The listing builds one solid part. Answer for the finished solid, in the listing's coordinates (mm). A direction names the side the tool comes from. Round coordinates to 2 decimals unless told otherwise and drop trailing zeros. Loops run counter-clockwise (first coordinate to the right, second up) from the corner with the lowest first, then second, coordinate; pieces in that order, holes last. Notation, with made-up numbers: (51, 61) -> (55, 61) arc R26 ccw to (55, 93) -> close; hole circle Ø6 at (12.25, 14.25). An arc over 180 degrees is marked (long way). Use a Markdown table: item, result. Add a question column.
Q1. Consider line 1 (Y direction, x = 0.1, z = -63.5); line 2 (Y direction, x = 1.25, z = -109); line 3 (Z direction, x = 1.85, y = -17.5). Determine where each line is inside the solid, lowest interval first.
Q2. Section B-B on y = -16.5 is taken. Give the vertices of the cut face in (x, z).
Q3. Section A-A on z = -14 is taken. Give the vertices of the cut face in (x, y), then the cut area to 3 significant figures.
Q4. For a pull along Y with two mould halves and no side action, classify faces 1 (the flat face through (1, 0, -65)), 2 (the flat face through (1.48, -44.61, -46.78)), 3 (the cylindrical face through (1.521, -11.014, -69.722)) as released by +Y, released by -Y, zero draft, split by the parting line, or undercut.
Q5. Which of the six approach directions +Z, -Z, +X, -X, +Y, -Y give full straight-line access (tool end or side, diameter ignored) to faces 4 (the flat face through (2, -9.884, -127)), 5 (the flat face through (1, -46, 0)), 6 (the flat face through (2, -36, -28.5))?
Q6. Given pin 1 Ø22.5 at (y, z) = (-35.05, -12.88) entering from -X; pin 2 Ø1.5 at (x, y) = (1.5, -46) entering from +Z, each flat-ended and moving along its own axis, determine where each tip first touches the part or whether it passes through.
Q7. Section C-C on z = -88 is taken. Give the vertices of the cut face in (x, y), then the cut area to 3 significant figures.
Q8. Section D-D on x = 2.05 is taken. Give the number of separate pieces and of enclosed holes in the cut face, then the cut area to 3 significant figures.
from build123d import *

# Parameters (mm, degrees)
BOSS_EXTRUDE1_DEPTH     = 3
SKETCH2_W               = 3
SKETCH2_H               = 28.023136596
SKETCH2_H_2             = 21.36601765
CUT_EXTRUDE1_DEPTH      = 20
SKETCH3_W               = 3
SKETCH3_H               = 30
BOSS_EXTRUDE2_DEPTH     = 3
SKETCH4_R               = 11.564612176
SKETCH4_R_2             = 9.45507824
SKETCH4_R_3             = 14.470802902
SKETCH4_R_4             = 9.678963713
SKETCH4_R_5             = 5.652740002
SKETCH4_R_6             = 5.531973284
SKETCH4_R_7             = 5.989913263
SKETCH4_R_8             = 6.729308726
SKETCH4_R_9             = 6.066934598
SKETCH4_R_10            = 6.829551901
CUT_EXTRUDE2_DEPTH      = 1
CUT_EXTRUDE2_DEPTH_BACK = 4
SKETCH5_W               = 3
SKETCH5_H               = 14
CUT_EXTRUDE3_DEPTH      = 10


with BuildPart() as part:
    # Sketch1 → Boss-Extrude1 (new body)
    with BuildSketch(Plane(origin=(0, 0, 0), x_dir=(0, 0, -1), z_dir=(1, 0, 0))):
        Polygon((0, 0), (0, -50.777676291), (129, -33.768874681), (129, 0), align=None)
    extrude(amount=BOSS_EXTRUDE1_DEPTH)

    # Sketch2 → Cut-Extrude1 (cut)
    with BuildSketch(Plane(origin=(3, 0, 0), x_dir=(0, 0, -1), z_dir=(1, 0, 0))):
        with Locations((30, -38.011568298)):
            Rectangle(SKETCH2_W, SKETCH2_H)
        with Locations((64, -34.683008825)):
            Rectangle(SKETCH2_W, SKETCH2_H_2)
    extrude(amount=-CUT_EXTRUDE1_DEPTH, mode=Mode.SUBTRACT)

    # Sketch3 → Boss-Extrude2 (add)
    with BuildSketch(Plane(origin=(3, 0, 0), x_dir=(0, 0, -1), z_dir=(1, 0, 0))):
        with Locations((-1.5, -25.777676291)):
            Rectangle(SKETCH3_W, SKETCH3_H)
    extrude(amount=-BOSS_EXTRUDE2_DEPTH)

    # Sketch4 → Cut-Extrude2 (cut, two sides)
    with BuildSketch(Plane(origin=(3, 0, 0), x_dir=(0, 0, -1), z_dir=(1, 0, 0))) as cut_extrude2_sk:
        with Locations((46.139822704, -19.984473783)):
            Circle(SKETCH4_R)
        with Locations((108.618953829, -10.917568804)):
            Circle(SKETCH4_R_2)
        with Locations((83.259777078, -19.984473783)):
            Circle(SKETCH4_R_3)
        with Locations((12.878873487, -12.542106693)):
            Circle(SKETCH4_R_4)
        with Locations((12.878873487, -35.052970113)):
            Circle(SKETCH4_R_4)
        with Locations((30.887564223, -7.517969022)):
            Circle(SKETCH4_R_5)
        with Locations((54.960405921, -36.18486448)):
            Circle(SKETCH4_R_6)
        with Locations((39.432504215, -38.114367059)):
            Circle(SKETCH4_R_7)
        with Locations((63.505345914, -8.436779774)):
            Circle(SKETCH4_R_8)
        with Locations((103.657375769, -28.650616315)):
            Circle(SKETCH4_R_9)
        with Locations((117.623299197, -26.537351586)):
            Circle(SKETCH4_R_10)
    extrude(amount=CUT_EXTRUDE2_DEPTH, mode=Mode.SUBTRACT)
    extrude(cut_extrude2_sk.sketch, amount=-CUT_EXTRUDE2_DEPTH_BACK, mode=Mode.SUBTRACT)

    # Sketch5 → Cut-Extrude3 (cut)
    with BuildSketch(Plane(origin=(3, 0, 0), x_dir=(0, 0, -1), z_dir=(1, 0, 0))):
        with Locations((127.5, -16.88443734)):
            Rectangle(SKETCH5_W, SKETCH5_H)
    extrude(amount=-CUT_EXTRUDE3_DEPTH, mode=Mode.SUBTRACT)


solid = part.part
Checked values:
| question | item | result |
|---|---|---|
| 1 | line 1 | y = -24 to -15.17, -1.71 to 0 |
| 1 | line 2 | y = -36.41 to -31.53, -25.78 to -20.36, -1.47 to 0 |
| 1 | line 3 | z = -126 to -115.41, -101.83 to -97.52, -69 to -57.43, -34.85 to -21.19, -4.57 to 3 |
| 2 | outline | (0, -126) -> (3, -126) -> (3, -116.25) -> (0, -116.25) -> close; (0, -100.99) -> (3, -100.99) -> (3, -97.3) -> (0, -97.3) -> close; (0, -69.21) -> (3, -69.21) -> (3, -57.17) -> (0, -57.17) -> close; (0, -35.11) -> (3, -35.11) -> (3, -21.71) -> (0, -21.71) -> close; (0, -4.05) -> (3, -4.05) -> (3, 3) -> (0, 3) -> close |
| 3 | outline | (0, -48.93) -> (3, -48.93) -> (3, -44.67) -> (0, -44.67) -> close; (0, -25.44) -> (3, -25.44) -> (3, -22.16) -> (0, -22.16) -> close; (0, -2.93) -> (3, -2.93) -> (3, 0) -> (0, 0) -> close |
| 3 | area | 31.4 mm2 |
| 4 | face 1 | released by +Y |
| 4 | face 2 | released by -Y |
| 4 | face 3 | undercut |
| 5 | face 4 | -Z, +X, -X |
| 5 | face 5 | +Z, +X, -X, -Y |
| 5 | face 6 | +X, -X, -Y |
| 6 | pin 1 | stops at x = 0 |
| 6 | pin 2 | stops at z = 0 |
| 7 | outline | (0, -39.17) -> (3, -39.17) -> (3, -33.66) -> (0, -33.66) -> close; (0, -6.31) -> (3, -6.31) -> (3, 0) -> (0, 0) -> close |
| 7 | area | 35.5 mm2 |
| 8 | separate pieces | 1 |
| 8 | enclosed holes | 11 |
| 8 | area | 2,720 mm2 |
